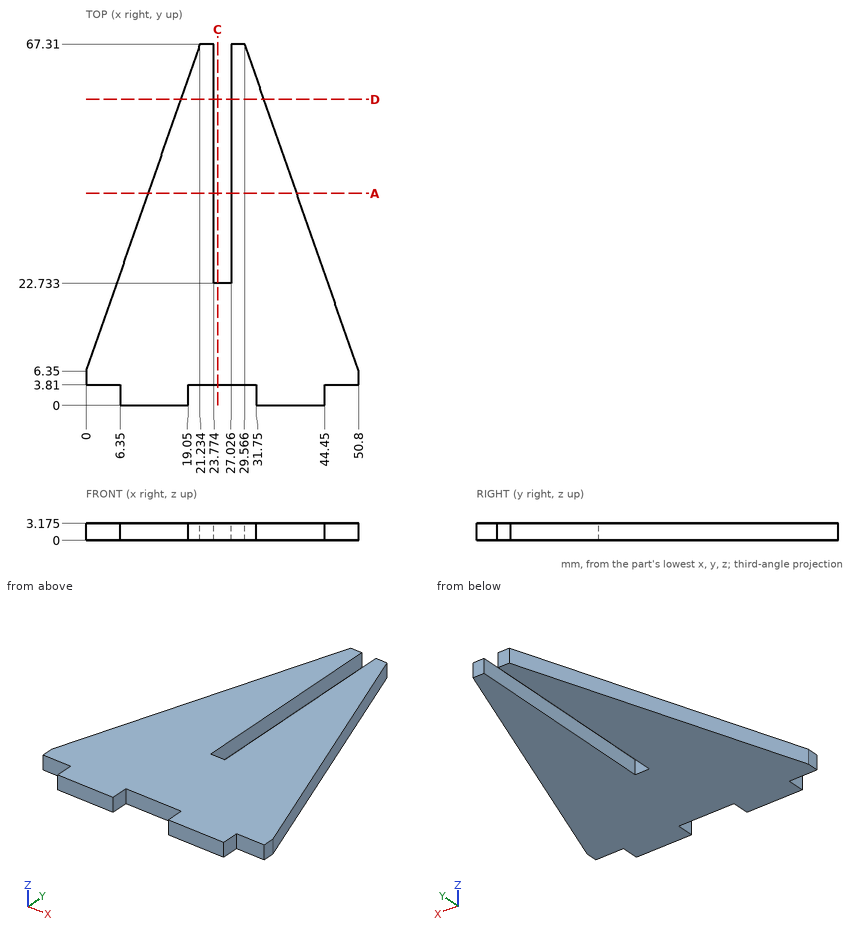
Input: dimensioned drawing with shaded views. Units: mm. Origin: part minimum x, y, z. Coordinates: 2 decimals unless noted, no trailing zeros. Order: outer loops, then holes, each group sorted by start corner. A loop starts at its lowest first (then second) coordinate and runs counter-clockwise, first axis right, second up. Notation, with made-up numbers: (12.25, -8.75) - (52.25, -8.75) arc R9 ccw to (52.25, -2.75) - close; hole circle Ø4 at (-9.5, -7.5). An arc over 180 degrees is marked (long way). Return JSON: item names as keys, results as strings. Group by question number.
1. Cut plane D-D (y = 57). Output: boundary loops of the cut face in (x, z) (1 decimal).
2. Cut plane A-A (y = 39.5). Output: boundary loops of the cut face in (x, z) (1 decimal).
3. Material intervals for line 1 along X through (y, z) = (47.5, 2.15) (1 decimal); line 2 along X through (y, z) = (60, 0.5) (1 decimal); line 3 along Y through (x, z) = (23.5, 2.2), sorted ascending. Write a range as [from, to].
4. Cut plane C-C (x = 24.5). Output: boundary loops of the cut face in (y, z) (1 decimal).
5. Pin query (flat end, axial travel): pin 1 (1.6 mm diameter, centred on y = 2.5, z = 2, fed in from -X); pin 2 (1.6 mm diameter, centred on x = 1.5, z = 1, fed in from -Y); pin 3 (1 mm diameter, centred on y = 37, z = 1.5, fed in from -X). Return the tip coordinate at first contact, or that it passes through.
Resolved:
{
 "1": {"outline": "(17.6, 0) - (23.8, 0) - (23.8, 3.2) - (17.6, 3.2) - close; (27, 0) - (33.2, 0) - (33.2, 3.2) - (27, 3.2) - close"},
 "2": {"outline": "(11.5, 0) - (23.8, 0) - (23.8, 3.2) - (11.5, 3.2) - close; (27, 0) - (39.3, 0) - (39.3, 3.2) - (27, 3.2) - close"},
 "3": {"line 1": "x = [14.3, 23.8], [27, 36.5]", "line 2": "x = [18.7, 23.8], [27, 32.1]", "line 3": "y = [3.81, 67.31]"},
 "4": {"outline": "(3.8, 0) - (22.7, 0) - (22.7, 3.2) - (3.8, 3.2) - close"},
 "5": {"pin 1": "stops at x = 6.35", "pin 2": "stops at y = 3.81", "pin 3": "stops at x = 10.5"}
}
